Can you work these out from the model? Positions are in its coordinate system, mm. A direction names the side the tool comes from. Give positions to 0.01 mm unless a question says otherwise; leave off trailing zeros. Write each loop counter-clockwise with the first axis right and the second up, starting at its lowest first coordinate (ties: lowest second). Pieces come first, ordered by that corner, then holes. Notation, with made-up numbers: M 1,-24.75 L 22,-24.75 A23 cw 22,-13.75 Z; hole C -27,24.5 d3. An arc over 180 degrees is marked long. Write each question's results on one line, items separated by ' | '.
from build123d import *

# Parameters (mm, degrees)
F1_DEPTH = 9.525
F6_R     = 5.08


with BuildPart() as f1:
    # F0 (on Top) → F1 (new body, symmetric)
    with BuildSketch(Plane.XY):
        with BuildLine():
            Line((0, 0), (0, -36.83))
            Line((0, -36.83), (7.62, -36.83))
            Line((7.62, -36.83), (7.62, -13.97))
            ThreePointArc((7.62, -13.97), (9.851846, -8.581846), (15.24, -6.35))
            Line((15.24, -6.35), (34.451012, -6.35))
            ThreePointArc((34.451012, -6.35), (35.558944, -6.374175), (36.664768, -6.446655))
            Line((36.664768, -6.446655), (101.84481, -12.149169))
            ThreePointArc((101.84481, -12.149169), (103.931366, -10.819887), (103.187418, -8.460385))
            Line((103.187418, -8.460385), (90.026374, 0.755077))
            Line((90.026374, 0.755077), (92.71, -4.999977))
            Line((92.71, -4.999977), (36.664768, -0.096655))
            ThreePointArc((36.664768, -0.096655), (35.558944, -0.024175), (34.451012, 0))
            Line((34.451012, 0), (15.24, 0))
            ThreePointArc((15.24, 0), (9.851846, 2.231846), (7.62, 7.62))
            Line((7.62, 7.62), (7.62, 10.16))
            Line((7.62, 10.16), (0, 10.16))
            Line((0, 10.16), (0, 0))
        make_face()
    extrude(amount=F1_DEPTH, both=True)

    # F2 (on Top) → F3 (revolve, cut)
    with BuildSketch(Plane.XY):
        Polygon((0, -19.05), (0, -20.701), (4.699, -20.701), (9.652, -24.85706), (11.555037, -24.85706), (11.555037, -19.05), (9.652, -19.05), align=None)
    revolve(axis=Axis((-2.504904, -19.05, 0), (-1, 0, 0)), mode=Mode.SUBTRACT)

    # F4 (on Top) → F5 (revolve, cut)
    with BuildSketch(Plane.XY):
        Polygon((7.62, -29.21), (0, -29.21), (0, -30.861), (5.08, -30.861), (7.62, -32.992313), align=None)
    revolve(axis=Axis((3.81, -29.21, 0), (1, 0, 0)), mode=Mode.SUBTRACT)

    # F6
    f6_edges = [f1.edges().sort_by_distance(p)[0] for p in [
        (3.81, -36.83, 9.525),
        (3.81, -36.83, -9.525),
    ]]
    fillet(f6_edges, radius=F6_R)

    # F7 (on Top) → F8 (revolve, cut)
    with BuildSketch(Plane.XY):
        Polygon((0, 5.08), (0, 3.429), (4.699, 3.429), (8.038316, 0.626982), (15.24, 0.626982), (15.24, 5.08), (8.038316, 5.08), align=None)
    revolve(axis=Axis((4.019158, 5.08, 0), (-1, 0, 0)), mode=Mode.SUBTRACT)


solid = f1.part
Item 1: I want a section at C-C, the plane y = -19.05. Please give me the cut outline in (x, z) (3 decimals).
Geometry says:
outline: M 0,-9.525 L 7.62,-9.525 L 7.62,-4.102 L 4.699,-1.651 L 0,-1.651 Z; M 0,1.651 L 4.699,1.651 L 7.62,4.102 L 7.62,9.525 L 0,9.525 Z
Item 2: I want a section at D-D, the plane x = 61. Please give me the cut outline in (y, z) (3 decimals).
Geometry says:
outline: M -8.576,-9.525 L -2.226,-9.525 L -2.226,9.525 L -8.576,9.525 Z
Item 3: If I drill on line 1 (Z direction, x = 3, y = -19) (3 decimals); line 2 (Z direction, x = 3, y = -29) (3 decimals); line 3 (X direction, y = -16, z = 7.75), over which ranges is the centre line in solid material (lowest first)? Write a range as from..to.
Geometry says:
line 1: z = -9.525..-1.65, 1.65..9.525 | line 2: z = -9.525..-1.638, 1.638..9.525 | line 3: x = 0..7.62
Item 4: I want a section at A-A, the plane y = -29.21. Please give me the cut outline in (x, z) (3 decimals).
Geometry says:
outline: M 0,-9.525 L 7.62,-9.525 L 7.62,-3.782 L 5.08,-1.651 L 0,-1.651 Z; M 0,1.651 L 5.08,1.651 L 7.62,3.782 L 7.62,9.525 L 0,9.525 Z
Item 5: Thinking about a two-plate mould opening in Z: for faces 5 (the face through (35.543, -6.374, 0.133)), 6 (the face through (9.69, 0.63, -0.1)), 7 (the face through (2.382, 3.555, -0.632)), 8 (the face through (3.86, -35.38, -8)), which applies, +Z half, -Z half, draft (parallel to the pull), parting line (faces both ways), or undercut?
Geometry says:
face 5: draft | face 6: undercut | face 7: undercut | face 8: -Z half
Item 6: For faces 1 (the face through (7.62, 9.4, 0.1)), 2 (the face through (7.62, -25.6, 2.3)), 3 (the face through (68.8, -9.26, 0.13)), 4 (the face through (12.096, 0.679, 2.25)), which set-ups out of +Z, -Z, +X, -X, +Y, -Y let a thin tool reach every point of the face, with its end or its side?
Geometry says:
face 1: +Z, -Z, +X, +Y | face 2: +Z, -Z, +X, -Y | face 3: +Z, -Z, -Y | face 4: +Z, -Z, +Y
Item 7: I'm going to push flat-ended pins straight in: pin 1 (4 mm diameter, centred on y = 5.08, z = 0, fed in from -X); pin 2 (9.5 mm diameter, centred on x = 24, z = 2.5, fed in from -Y); pin 3 (1.5 mm diameter, centred on x = 92, z = 7, fed in from -Y); pin 4 (1 mm diameter, centred on x = 79, z = 1.5, fed in from +Y). Where does each tip first touch, or does it pass through?
Geometry says:
pin 1: stops at x = 0 | pin 2: stops at y = -6.35 | pin 3: stops at y = -11.35 | pin 4: stops at y = -3.76
Item 8: I want a section at B-B, the plane z = 0. Give the number of separate pieces and of enclosed holes in the cut face, and give its area (3 significant figures).
Geometry says:
separate pieces: 4 | enclosed holes: 0 | area: 900 mm2
